Input: part model. Units: mm. Frame: model coordinates. Round coordinates to 2 decimals unless told otherwise and drop trailing zeros. Write each loop counter-clockwise with the first axis right and the second up, starting at its lowest first coordinate (ties: lowest second). Pieces come first, ordered by that corner, then holes. Notation, with made-up numbers: (-37, 27) - (0, 27) arc R33 cw to (0, 57) - close; hole circle Ø10 at (75, 83.5). An arc over 180 degrees is marked (long way). Use one line per item in the form item = value.
```python
from build123d import *

# Parameters (mm, degrees)
SKICA2_W                 = 29.8
SKICA2_H                 = 4.2
P_IDAT_VYSUNUT_M2_DEPTH  = 0.4
SKICA3_R                 = 1.75
P_IDAT_VYSUNUT_M3_DEPTH  = 1.5
SKICA5_R                 = 1.9
P_IDAT_VYSUNUT_M5_DEPTH  = 2
ZKOSEN_2_SIZE            = 1.5
SKICA7_W                 = 1
SKICA7_H                 = 5
ODEBRAT_VYSUNUT_M1_DEPTH = 3.5
SKICA8_W                 = 4.2
SKICA8_H                 = 24.8
P_IDAT_VYSUNUT_M6_DEPTH  = 0.4
SKICA9_R                 = 1.75
P_IDAT_VYSUNUT_M7_DEPTH  = 1.5
SKICA10_R                = 1.9
P_IDAT_VYSUNUT_M8_DEPTH  = 2
ZKOSEN_3_SIZE            = 1.5
SKICA12_W                = 5
SKICA12_H                = 1
ODEBRAT_VYSUNUT_M2_DEPTH = 3.5
ZAOBLIT1_R               = 15
ZAOBLIT2_R               = 20


with BuildPart() as part:
    # Skica2 → Přidat vysunutím2 (new body)
    with BuildSketch(Plane.XY):
        Rectangle(SKICA2_W, SKICA2_H)
    extrude(amount=P_IDAT_VYSUNUT_M2_DEPTH)

    # Skica3 → Přidat vysunutím3 (add)
    with BuildSketch(Plane.XY.offset(0.4)):
        with Locations((7.9, 0)):
            Circle(SKICA3_R)
    extrude(amount=P_IDAT_VYSUNUT_M3_DEPTH)

    # Skica5 → Přidat vysunutím5 (add)
    with BuildSketch(Plane.XY.offset(1.9)):
        with Locations((7.9, 0)):
            Circle(SKICA5_R)
    extrude(amount=P_IDAT_VYSUNUT_M5_DEPTH)

    # Zkosení2
    zkosen_2_edges = [part.edges().sort_by_distance(p)[0] for p in [
        (6, 0, 3.9),
    ]]
    chamfer(zkosen_2_edges, length=ZKOSEN_2_SIZE)

    # Skica7 → Odebrat vysunutím1 (cut)
    with BuildSketch(Plane.XY.offset(3.9)):
        with Locations((7.9, 0)):
            Rectangle(SKICA7_W, SKICA7_H)
    extrude(amount=-ODEBRAT_VYSUNUT_M1_DEPTH, mode=Mode.SUBTRACT)

    # Skica8 → Přidat vysunutím6 (add)
    with BuildSketch(Plane(origin=(0, 0, 0), x_dir=(-1, 0, 0), z_dir=(0, 0, -1))):
        with Locations((12.8, -14.5)):
            Rectangle(SKICA8_W, SKICA8_H)
    extrude(amount=-P_IDAT_VYSUNUT_M6_DEPTH)

    # Skica9 → Přidat vysunutím7 (add)
    with BuildSketch(Plane.XY.offset(0.4)):
        with Locations((-12.8, -19.9)):
            Circle(SKICA9_R)
    extrude(amount=P_IDAT_VYSUNUT_M7_DEPTH)

    # Skica10 → Přidat vysunutím8 (add)
    with BuildSketch(Plane.XY.offset(1.9)):
        with Locations((-12.8, -19.9)):
            Circle(SKICA10_R)
    extrude(amount=P_IDAT_VYSUNUT_M8_DEPTH)

    # Zkosení3
    zkosen_3_edges = [part.edges().sort_by_distance(p)[0] for p in [
        (-14.7, -19.9, 3.9),
    ]]
    chamfer(zkosen_3_edges, length=ZKOSEN_3_SIZE)

    # Skica12 → Odebrat vysunutím2 (cut)
    with BuildSketch(Plane.XY.offset(3.9)):
        with Locations((-12.8, -19.9)):
            Rectangle(SKICA12_W, SKICA12_H)
    extrude(amount=-ODEBRAT_VYSUNUT_M2_DEPTH, mode=Mode.SUBTRACT)

    # Zaoblit1
    zaoblit1_edges = [part.edges().sort_by_distance(p)[0] for p in [
        (-10.7, -2.1, 0.2),
    ]]
    fillet(zaoblit1_edges, radius=ZAOBLIT1_R)

    # Zaoblit2
    zaoblit2_edges = [part.edges().sort_by_distance(p)[0] for p in [
        (-14.9, 2.1, 0.2),
    ]]
    fillet(zaoblit2_edges, radius=ZAOBLIT2_R)


solid = part.part
```
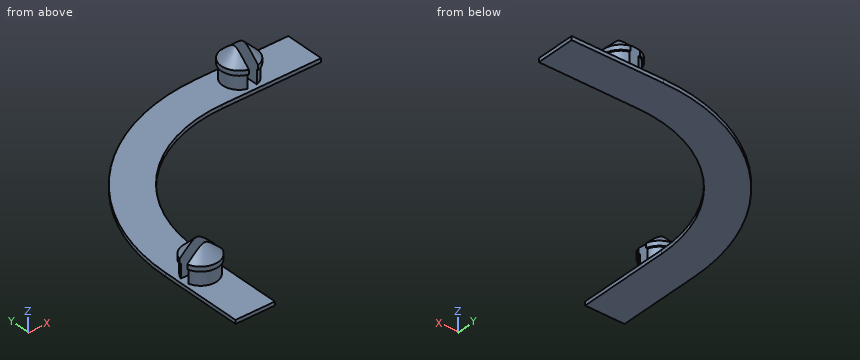
(1) Cut plane A-A on z = 1.55. Output: boundary loops of the cut face in (x, y), then the cut area to 3 significant figures.
Derived:
outline = (-14.48, -20.4) arc R1.75 ccw to (-11.12, -20.4) - close; (-14.48, -19.4) - (-11.12, -19.4) arc R1.75 ccw to start; (7.4, -1.68) - (7.4, 1.68) arc R1.75 ccw to start; (8.4, -1.68) arc R1.75 ccw to (8.4, 1.68) - close
area = 12.3 mm^2
(2) Material intervals for L1, parallel to Z at x = -11.5, y = -7.25; L2, parallel to Y at x = -12, z = 2.6; L3, parallel to Z at x = 9, y = -1.5, sorted ascending.
Derived:
L1 = 0 to 0.4
L2 = -21.4 to -20.4, -19.4 to -18.4
L3 = 0 to 0.4, 1.9 to 2.44
(3) Cut plane B-B on x = 11.5. Output: boundary loops of the cut face in (y, z), then the cut area to 3 significant figures.
Derived:
outline = (-2.1, 0) - (2.1, 0) - (2.1, 0.4) - (-2.1, 0.4) - close
area = 1.68 mm^2
(4) Cut plane C-C on z = 3.3. Output: boundary loops of the cut face in (x, y), then the cut area to 3 significant figures.
Derived:
outline = (-13.67, -20.4) arc R1 ccw to (-11.93, -20.4) - close; (-13.67, -19.4) - (-11.93, -19.4) arc R1 ccw to start; (7.4, -0.87) - (7.4, 0.87) arc R1 ccw to start; (8.4, -0.87) arc R1 ccw to (8.4, 0.87) - close
area = 2.46 mm^2
(5) Cut plane D-D on y = -19.75. Output: boundary loops of the cut face in (x, z), then the cut area to 3 significant figures.
Derived:
outline = (-14.9, 0) - (-10.7, 0) - (-10.7, 0.4) - (-14.9, 0.4) - close
area = 1.68 mm^2
(6) First-contact query: pin 1 Ø1.5 at (x, z) = (9.5, 1.5) entering from -Y; pin 2 Ø1.7 at (x, z) = (-13, 2) entering from -Y; pin 3 Ø1 at (y, z) = (0.5, 1.5) entering from +X; pin 4 Ø1.5 at (y, z) = (-15, 2.5) entering from +X. Flat tips, straight axial feed; report the tip coordinate or a pass-through.
Derived:
pin_1 = -1.64
pin_2 = -21.8
pin_3 = 9.79
pin_4 = through
